from build123d import *

# Parameters (mm, degrees)
SKETCH1_W           = 100
SKETCH1_H           = 98
SKETCH1_W_2         = 40.347954038
SKETCH1_H_2         = 3
SKETCH1_W_3         = 96
SKETCH1_W_4         = 40.652045962
SKETCH1_R           = 5
BOSS_EXTRUDE4_DEPTH = 3
SKETCH1_8_W         = 6
SKETCH1_8_H         = 6
SKETCH1_8_R         = 1.5
BOSS_EXTRUDE6_DEPTH = 4
FILLET3_R           = 4


with BuildPart() as part:
    # Sketch1 → Boss-Extrude4 (new body)
    with BuildSketch(Plane(origin=(0, 0, 0), x_dir=(1, 0, 0), z_dir=(0, 1, 0))):
        Rectangle(SKETCH1_W, SKETCH1_H)
        with Locations((-27.826022981, -4.136363636)):
            Rectangle(SKETCH1_W_2, SKETCH1_H_2, mode=Mode.SUBTRACT)
        with Locations((0, -45.5)):
            Rectangle(SKETCH1_W_3, SKETCH1_H_2, mode=Mode.SUBTRACT)
        with Locations((0, -37.227272727)):
            Rectangle(SKETCH1_W_3, SKETCH1_H_2, mode=Mode.SUBTRACT)
        with Locations((0, -28.954545455)):
            Rectangle(SKETCH1_W_3, SKETCH1_H_2, mode=Mode.SUBTRACT)
        with Locations((0, -20.681818182)):
            Rectangle(SKETCH1_W_3, SKETCH1_H_2, mode=Mode.SUBTRACT)
        with Locations((0, -12.409090909)):
            Rectangle(SKETCH1_W_3, SKETCH1_H_2, mode=Mode.SUBTRACT)
        with Locations((27.673977019, -4.136363636)):
            Rectangle(SKETCH1_W_4, SKETCH1_H_2, mode=Mode.SUBTRACT)
        with Locations((-27.826022981, 4.136363636)):
            Rectangle(SKETCH1_W_2, SKETCH1_H_2, mode=Mode.SUBTRACT)
        with Locations((0, 12.409090909)):
            Rectangle(SKETCH1_W_3, SKETCH1_H_2, mode=Mode.SUBTRACT)
        with Locations((0, 20.681818182)):
            Rectangle(SKETCH1_W_3, SKETCH1_H_2, mode=Mode.SUBTRACT)
        with Locations((0, 28.954545455)):
            Rectangle(SKETCH1_W_3, SKETCH1_H_2, mode=Mode.SUBTRACT)
        with Locations((0, 37.227272727)):
            Rectangle(SKETCH1_W_3, SKETCH1_H_2, mode=Mode.SUBTRACT)
        with Locations((0, 45.5)):
            Rectangle(SKETCH1_W_3, SKETCH1_H_2, mode=Mode.SUBTRACT)
        with Locations(Location((-0.152045962, 0, 0), (0, 0, 270))):
            Circle(SKETCH1_R, mode=Mode.SUBTRACT)
        with Locations((27.673977019, 4.136363636)):
            Rectangle(SKETCH1_W_4, SKETCH1_H_2, mode=Mode.SUBTRACT)
    extrude(amount=BOSS_EXTRUDE4_DEPTH)

    # Sketch1_8 → Boss-Extrude6 (add)
    # profile 1 of 4: a face of its own
    with BuildSketch(Plane(origin=(0, 0, 0), x_dir=(1, 0, 0), z_dir=(0, 1, 0))):
        with Locations((-47, -52)):
            Rectangle(SKETCH1_8_W, SKETCH1_8_H)
        with Locations(Location((-47, -52, 0), (0, 0, 270))):
            Circle(SKETCH1_8_R, mode=Mode.SUBTRACT)
    # profile 2 of 4: a face of its own
    with BuildSketch(Plane(origin=(0, 0, 0), x_dir=(1, 0, 0), z_dir=(0, 1, 0))):
        with Locations((47, -52)):
            Rectangle(SKETCH1_8_W, SKETCH1_8_H)
        with Locations(Location((47, -52, 0), (0, 0, 270))):
            Circle(SKETCH1_8_R, mode=Mode.SUBTRACT)
    # profile 3 of 4: a face of its own
    with BuildSketch(Plane(origin=(0, 0, 0), x_dir=(1, 0, 0), z_dir=(0, 1, 0))):
        with Locations((47, 52)):
            Rectangle(SKETCH1_8_W, SKETCH1_8_H)
        with Locations(Location((47, 52, 0), (0, 0, 270))):
            Circle(SKETCH1_8_R, mode=Mode.SUBTRACT)
    # profile 4 of 4: a face of its own
    with BuildSketch(Plane(origin=(0, 0, 0), x_dir=(1, 0, 0), z_dir=(0, 1, 0))):
        with Locations((-47, 52)):
            Rectangle(SKETCH1_8_W, SKETCH1_8_H)
        with Locations(Location((-47, 52, 0), (0, 0, 270))):
            Circle(SKETCH1_8_R, mode=Mode.SUBTRACT)
    extrude(amount=BOSS_EXTRUDE6_DEPTH)

    # Fillet3
    fillet3_edges = [part.edges().sort_by_distance(p)[0] for p in [
        (-44, 1.5, 49),
        (44, 1.5, 49),
        (44, 1.5, -49),
        (-44, 1.5, -49),
    ]]
    fillet(fillet3_edges, radius=FILLET3_R)


solid = part.part
CAD build for the part. Positions are in the model's coordinates, mm. A direction names the side the tool comes from. Coordinates: 2 decimals unless noted, no trailing zeros. Answer as a JSON object with one key per item and string values. Group by question number.
1) Pin check, flat tips, straight feed: pin 1 Ø3 at (x, z) = (-35, 30) entering from +Y; pin 2 Ø0.9 at (x, y) = (15, 2) entering from +Z; pin 3 Ø0.9 at (x, y) = (12.5, 2) entering from -Z. Stop position of each tip, or through.
2) Tool access for faces 4 (the face through (-1, 1, 13.909)), 5 (the face through (42.859, 1.521, 50.203)): list every direction of +Z, -Z, +X, -X, +Y, -Y with a clear straight run to the whole face (end or side of a thin tool).
3) Saw through at A-A (x = 24.5). Give the number of separate pieces and of enclosed holes in the cut face, plus the area to 3 significant figures.
4) Mould opens along Z. For faces 1 (the face through (-47, 2, -55)), 2 (the face through (50, 2, 1)), 3 (the face through (-7.652, 1, 4)) say: +Z half, -Z half, draft (parallel to the pull), parting line (faces both ways), or undercut.
5) Wall check: line 1 (X direction, y = 1.35, z = 52); line 2 (Y direction, x = 19, z = 25). Give the ranges that are in metal, low to high. Write a range as from..to.
Values follow:
{
 "1": {"pin 1": "stops at y = 3", "pin 2": "stops at z = 49", "pin 3": "stops at z = -49"},
 "2": {"face 4": "+Y, -Y", "face 5": "+Z, +Y, -Y"},
 "3": {"separate pieces": "13", "enclosed holes": "0", "area": "186 mm2"},
 "4": {"face 1": "-Z half", "face 2": "draft", "face 3": "undercut"},
 "5": {"line 1": "x = -50..-48.5, -45.5..-43.87, 43.87..45.5, 48.5..50", "line 2": "y = 0..3"}
}
